```python
from build123d import *

# Parameters (mm, degrees)
SKETCH1_W          = 50
SKETCH1_H          = 50
SKETCH1_W_2        = 46
SKETCH1_H_2        = 46
STEELTUBE_DEPTH    = 414
SKETCH2_R          = 4
CUT_EXTRUDE1_DEPTH = 2


with BuildPart() as part:
    # Sketch1 → steelTube (new body)
    with BuildSketch(Plane.XY):
        with Locations((-23, 23)):
            Rectangle(SKETCH1_W, SKETCH1_H)
        with Locations((-23, 23)):
            Rectangle(SKETCH1_W_2, SKETCH1_H_2, mode=Mode.SUBTRACT)
    extrude(amount=STEELTUBE_DEPTH)

    # Sketch2 → Cut-Extrude1 (cut)
    with BuildSketch(Plane.XZ.offset(2)):
        with Locations((-23, 50.3)):
            Circle(SKETCH2_R)
        with Locations((-23, 397.3)):
            Circle(SKETCH2_R)
    extrude(amount=-CUT_EXTRUDE1_DEPTH, mode=Mode.SUBTRACT)


solid = part.part
```
Could you check a few things on this model? Use its own coordinates, in mm. A direction names the side the tool comes from. Coordinates: 2 decimals unless noted, no trailing zeros. Loops run counter-clockwise (first coordinate to the right, second up) from the corner with the lowest first, then second, coordinate; pieces in that order, holes last.
1) Please list where these lines run through material, in increasing order: line 1 along Z through (x, y) = (-23, -1); line 2 along X through (y, z) = (2, 94.5); line 3 along Y through (x, z) = (-35, 58.5).
Reported:
line 1: z = 0 to 46.3, 54.3 to 393.3, 401.3 to 414
line 2: x = -48 to -46, 0 to 2
line 3: y = -2 to 0, 46 to 48
2) Imagine slicing it at C-C (z = 235.5). List the corners of the cut face in (x, y) for me.
Reported:
outline: (-48, -2) - (2, -2) - (2, 48) - (-48, 48) - close; hole (-46, 0) - (0, 0) - (0, 46) - (-46, 46) - close
3) Imagine slicing it at A-A (x = -23). List the corners of the cut face in (y, z) for me, and give its area (3 significant figures).
Reported:
outline: (-2, 0) - (0, 0) - (0, 46.3) - (-2, 46.3) - close; (-2, 54.3) - (0, 54.3) - (0, 393.3) - (-2, 393.3) - close; (-2, 401.3) - (0, 401.3) - (0, 414) - (-2, 414) - close; (46, 0) - (48, 0) - (48, 414) - (46, 414) - close
area: 1,620 mm2
4) Will these pins go through, and if not, where does the flat tip stop? pin 1 Ø5 at (x, z) = (-23, 50.3) entering from -Y; pin 2 Ø12 at (x, y) = (-38, 7) entering from -Z.
Reported:
pin 1: stops at y = 46
pin 2: passes through
5) Imagine slicing it at B-B (y = 30). List the corners of the cut face in (x, z) for me.
Reported:
outline: (-48, 0) - (-46, 0) - (-46, 414) - (-48, 414) - close; (0, 0) - (2, 0) - (2, 414) - (0, 414) - close
6) Which directions (+Z, -Z, +X, -X, +Y, -Y) give clear straight access to the entire face, cutting with the end or side of a thin tool? Please do faces 1 (the face through (-23, 48, 204)), 2 (the face through (-23.521, -1.014, 401.266)), 3 (the face through (0, 23, 204)).
Reported:
face 1: +Z, -Z, +X, -X, +Y
face 2: -Y
face 3: +Z, -Z
7) Thinking about a two-plate mould opening in Z: for faces 4 (the face through (2, 23, 204)), 5 (the face through (-23.521, -1.014, 54.266)), 6 (the face through (-25, -1, 0)), which applies, released by +Z, released by -Z, zero draft, split by the parting line, or undercut?
Reported:
face 4: zero draft
face 5: undercut
face 6: released by -Z
8) Imagine slicing it at D-D (x = -7). List the corners of the cut face in (y, z) for me, and give its area (3 significant figures).
Reported:
outline: (-2, 0) - (0, 0) - (0, 414) - (-2, 414) - close; (46, 0) - (48, 0) - (48, 414) - (46, 414) - close
area: 1,660 mm2
